The listing builds one solid part. Answer for the finished solid, in the listing's coordinates (mm). Give positions to 0.01 mm unless a question says otherwise; leave off trailing zeros. Order: outer loops, then holes, each group sorted by start corner. A loop starts at its lowest first (then second) coordinate and runs counter-clockwise, first axis right, second up. Notation, with made-up numbers: (59.25, 46.5) - (66.25, 46.5) arc R22 cw to (66.25, 59.5) - close; hole circle Ø7 at (8.25, -27.75). An arc over 180 degrees is marked (long way). Answer in a Markdown table with one row per item.
from build123d import *

# Parameters (mm, degrees)
SKETCH1_R           = 15.75
SKETCH1_R_2         = 1.6
BOSS_EXTRUDE2_DEPTH = 1.5


with BuildPart() as part:
    # Sketch1 → Boss-Extrude2 (new body)
    with BuildSketch(Plane(origin=(0, 0, 0), x_dir=(1, 0, 0), z_dir=(0, 1, 0))):
        with BuildLine():
            Line((-17.890919225, 47.151235704), (29.109080775, 47.151235704))
            ThreePointArc((29.109080775, 47.151235704), (31.230401119, 46.272556047), (32.109080775, 44.151235704))
            Line((32.109080775, 44.151235704), (32.109080775, -15.848764296))
            ThreePointArc((32.109080775, -15.848764296), (31.230401119, -17.97008464), (29.109080775, -18.848764296))
            Line((29.109080775, -18.848764296), (-17.890919225, -18.848764296))
            ThreePointArc((-17.890919225, -18.848764296), (-20.012239568, -17.97008464), (-20.890919225, -15.848764296))
            Line((-20.890919225, -15.848764296), (-20.890919225, 44.151235704))
            ThreePointArc((-20.890919225, 44.151235704), (-20.012239568, 46.272556047), (-17.890919225, 47.151235704))
        make_face()
        with Locations(Location((6.109080775, 1.151235704, 0), (0, 0, 270))):
            Circle(SKETCH1_R, mode=Mode.SUBTRACT)
        with Locations(Location((28.909080775, 22.151235704, 0), (0, 0, 270))):
            Circle(SKETCH1_R_2, mode=Mode.SUBTRACT)
    extrude(amount=BOSS_EXTRUDE2_DEPTH)


solid = part.part
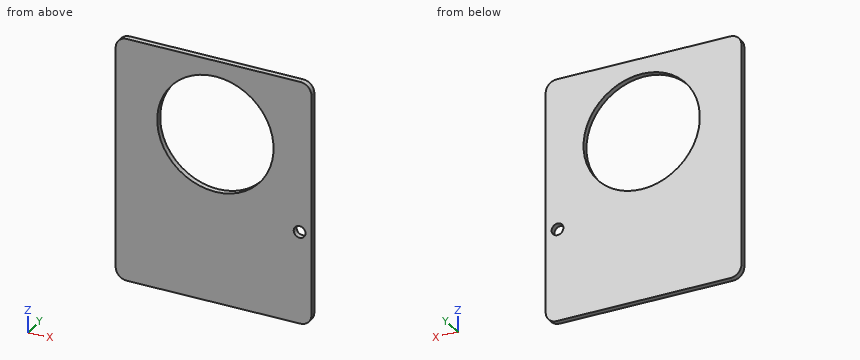
Item 1: This flat-tipped pin is pushed along its axis until it touches: P1, Ø3, axis at x = 28.91, z = -22.15, coming from the -Y side. Where does it stop, or does it pass through?
Answer block:
| item | result |
|---|---|
| P1 | through |
Item 2: Consider line 1 (X direction, y = 0.25, z = -1); line 2 (X direction, y = 0.1, z = -8); line 3 (Z direction, x = -7.5, y = 1.35). Determine where each line is inside the solid, lowest interval first.
Answer block:
| item | result |
|---|---|
| line 1 | -20.89 to -9.64, 21.86 to 32.11 |
| line 2 | -20.89 to -8.07, 20.29 to 32.11 |
| line 3 | -47.15 to -9.08, 6.78 to 18.85 |
Item 3: Find section C-C on y = 0.35. Write down the section's boundary in (x, z), then the cut area to 3 significant figures.
Answer block:
| item | result |
|---|---|
| outline | (-20.89, -44.15) arc R3 ccw to (-17.89, -47.15) - (29.11, -47.15) arc R3 ccw to (32.11, -44.15) - (32.11, 15.85) arc R3 ccw to (29.11, 18.85) - (-17.89, 18.85) arc R3 ccw to (-20.89, 15.85) - close; hole circle Ø31.5 at (6.11, -1.15); hole circle Ø3.2 at (28.91, -22.15) |
| area | 2,700 mm² |
Item 4: Find section B-B on x = 15.5. Write down the section's boundary in (y, z).
Answer block:
| item | result |
|---|---|
| outline | (0, -47.15) - (1.5, -47.15) - (1.5, -13.8) - (0, -13.8) - close; (0, 11.49) - (1.5, 11.49) - (1.5, 18.85) - (0, 18.85) - close |
Item 5: Find section A-A on z = 0. Write down the section's boundary in (x, y).
Answer block:
| item | result |
|---|---|
| outline | (-20.89, 0) - (-9.6, 0) - (-9.6, 1.5) - (-20.89, 1.5) - close; (21.82, 0) - (32.11, 0) - (32.11, 1.5) - (21.82, 1.5) - close |
